```python
from build123d import *

# Parameters (mm, degrees)
F1_DEPTH = 88.9
F2_R     = 3.175
F3_DEPTH = 25.4
F4_R     = 3.175
F5_DEPTH = 25.4


with BuildPart() as f1:
    # F0 (on Front) → F1 (new body)
    with BuildSketch(Plane.XZ):
        Polygon((-57.892904, 8.5725), (-57.892904, -29.5275), (-51.542904, -29.5275), (-51.542904, 2.2225), (202.457096, 2.2225), (202.457096, 8.5725), align=None)
    extrude(amount=F1_DEPTH)

    # F2 (on face) → F3 (cut)
    with BuildSketch(Plane.XY.offset(8.5725)):
        with Locations((119.907096, -63.1698)):
            Circle(F2_R)
        with Locations((119.907096, -48.8696)):
            Circle(F2_R)
        with Locations((186.607496, -63.1698)):
            Circle(F2_R)
        with Locations((186.607496, -48.8696)):
            Circle(F2_R)
    extrude(amount=-F3_DEPTH, mode=Mode.SUBTRACT)

    # F4 (on face) → F5 (cut)
    with BuildSketch(Plane(origin=(-57.892904, 0, 0), x_dir=(0, -1, 0), z_dir=(-1, 0, 0))):
        with Locations((12.7, -16.8275)):
            Circle(F4_R)
        with Locations((76.2, -16.8275)):
            Circle(F4_R)
    extrude(amount=-F5_DEPTH, mode=Mode.SUBTRACT)


solid = f1.part
```
The listing builds one solid part. Answer for the finished solid, in the listing's coordinates (mm). A direction names the side the tool comes from. Coordinates: 2 decimals unless noted, no trailing zeros. Write each loop counter-clockwise with the first axis right and the second up, starting at its lowest first coordinate (ties: lowest second). Pieces come first, ordered by that corner, then holes. Notation, with made-up numbers: M 80,88.25 L 137,88.25 A25 ccw 137,100.25 Z; hole C -23.75,49.5 d8. An arc over 180 degrees is marked long. Use a Markdown table: item, result. Add a question column.
1. For a pull along Y with two mould halves and no side action, classify faces 3 (the flat face through (202.457, -44, 5)), 4 (the flat face through (52, 0, 4)), 5 (the cylindrical face through (184.088, -50.802, 5.442)), 6 (the cylindrical face through (117.388, -65.102, 5.442)) as +Y half, -Y half, draft (parallel to the pull), parting line (faces both ways), or undercut.
2. Section B-B (y = -70) is taken. Give the vertices of the cut face in (x, z), plus the area to 3 significant figures.
3. Given P1, Ø5, axis at x = 186.61, y = -48.87, coming from the +Z side; P2, Ø10, axis at x = 119.91, y = -48.87, coming from the -Z side; P3, Ø8, axis at y = -20.5, z = -25.5, coming from the +X side, each flat-ended and moving along its own axis, determine where each tip first touches the part or whether it passes through.
4. Section C-C (z = 0) is taken. Give the vertices of the cut face in (x, y), plus the area to 3 significant figures.
5. Straight lines are drawn through the part: line 1 along Z through (x, y) = (-56.25, -12.7); line 2 along Z through (x, y) = (35, -47); line 3 along X through (y, z) = (-44, -25.5). For each, find the intervals that lie inside material, in ascending order. Write a range as [from, to].
6. Section A-A (y = -12.7) is taken. Give the vertices of the cut face in (x, z).
7. Section D-D (x = 74.5) is taken. Give the vertices of the cut face in (y, z).
8. Which of the six approach directions +Z, -Z, +X, -X, +Y, -Y give full straight-line access (tool end or side, diameter ignored) to faces 1 (the flat face through (-51.543, -44, -14)), 2 (the cylindrical face through (-54.76, -77.67, -19.64))?
Data:
| question | item | result |
|---|---|---|
| 1 | face 3 | draft |
| 1 | face 4 | +Y half |
| 1 | face 5 | undercut |
| 1 | face 6 | undercut |
| 2 | outline | M -57.89,-29.53 L -51.54,-29.53 L -51.54,2.22 L 202.46,2.22 L 202.46,8.57 L -57.89,8.57 Z |
| 2 | area | 1,850 mm2 |
| 3 | P1 | passes through |
| 3 | P2 | stops at z = 2.22 |
| 3 | P3 | stops at x = -51.54 |
| 4 | outline | M -57.89,-88.9 L -51.54,-88.9 L -51.54,0 L -57.89,0 Z |
| 4 | area | 565 mm2 |
| 5 | line 1 | z = [-29.53, -20], [-13.65, 8.57] |
| 5 | line 2 | z = [2.22, 8.57] |
| 5 | line 3 | x = [-57.89, -51.54] |
| 6 | outline | M -57.89,-29.53 L -51.54,-29.53 L -51.54,-20 L -57.89,-20 Z; M -57.89,-13.65 L -51.54,-13.65 L -51.54,2.22 L 202.46,2.22 L 202.46,8.57 L -57.89,8.57 Z |
| 7 | outline | M -88.9,2.22 L 0,2.22 L 0,8.57 L -88.9,8.57 Z |
| 8 | face 1 | -Z, +X, +Y, -Y |
| 8 | face 2 | +X, -X |
